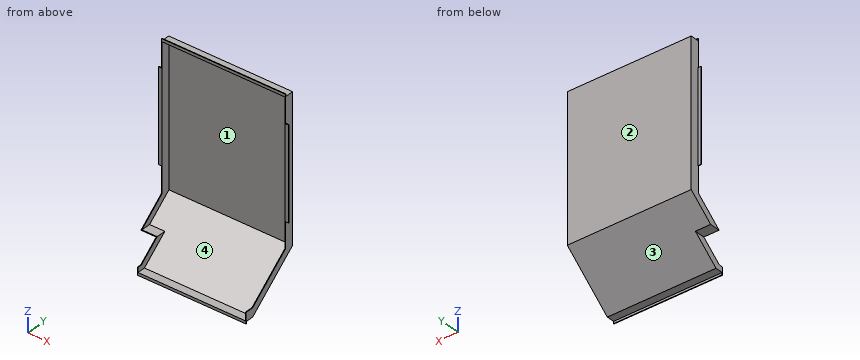
```python
from build123d import *

# Parameters (mm, degrees)
BOSS_EXTRUDE1_DEPTH  = 203
SKETCH4_W            = 2
SKETCH4_H            = 467.122613679
BOSS_EXTRUDE4_DEPTH  = 27
SKETCH5_W            = 2
SKETCH5_H            = 209.8319636
BOSS_EXTRUDE5_DEPTH  = 20
SKETCH6_W            = 2
SKETCH6_H            = 26.5
BOSS_EXTRUDE6_DEPTH  = 26.5
SKETCH14_W           = 300
SKETCH14_H           = 2
BOSS_EXTRUDE10_DEPTH = 10
SKETCH8_W            = 50
SKETCH8_H            = 77
CUT_EXTRUDE1_DEPTH   = 189.24061
BOSS_EXTRUDE7_DEPTH  = 48
SKETCH11_W           = 2
SKETCH11_H           = 107.789220226
BOSS_EXTRUDE8_DEPTH  = 20
CUT_EXTRUDE2_DEPTH   = 2
SKETCH13_W           = 2
SKETCH13_H           = 26.5
BOSS_EXTRUDE9_DEPTH  = 15.320889


with BuildPart() as part:
    # Sketch2 → Boss-Extrude1 (new body)
    with BuildSketch(Plane(origin=(0, 0, 0), x_dir=(0, 0, -1), z_dir=(1, 0, 0))):
        Polygon((-49.538744354, 1.5), (-49.538744354, -25.5), (-58.538744354, -25.5), (-58.538744354, -23.5), (-51.538744354, -23.5), (-51.538744354, 3.5), (418.516484641, 3.5), (554.461255643, -158.512669236), (554.461255643, -183.740609705), (561.461255643, -183.740609705), (561.461255643, -185.740609705), (552.461255643, -185.740609705), (552.461255643, -159.240609705), (417.583869325, 1.5), align=None)
    boss_extrude1 = extrude(amount=BOSS_EXTRUDE1_DEPTH)

    # Sketch4 → Boss-Extrude4 (add)
    with BuildSketch(Plane(origin=(0, 1.5, 0), x_dir=(-1, 0, 0), z_dir=(0, -1, 0))):
        with Locations((-202, 184.022562486)):
            Rectangle(SKETCH4_W, SKETCH4_H)
    boss_extrude4 = extrude(amount=BOSS_EXTRUDE4_DEPTH)

    # Sketch5 → Boss-Extrude5 (add)
    with BuildSketch(Plane(origin=(0, 206.239679889, -245.786879443), x_dir=(1, 0, 0), z_dir=(0, -0.6427876096865444, 0.7660444431189738))):
        with Locations((202, -372.184652342)):
            Rectangle(SKETCH5_W, SKETCH5_H)
    boss_extrude5 = extrude(amount=BOSS_EXTRUDE5_DEPTH)

    # Sketch6 → Boss-Extrude6 (add)
    with BuildSketch(Plane.XY.offset(-552.461255643)):
        with Locations((202, -172.490609705)):
            Rectangle(SKETCH6_W, SKETCH6_H)
    boss_extrude6 = extrude(amount=BOSS_EXTRUDE6_DEPTH)

    # Sketch14 → Boss-Extrude10 (add)
    with BuildSketch(Plane(origin=(203, 0, 0), x_dir=(0, 0, -1), z_dir=(1, 0, 0))):
        with Locations((181.461255646, -24.5)):
            Rectangle(SKETCH14_W, SKETCH14_H)
    boss_extrude10 = extrude(amount=BOSS_EXTRUDE10_DEPTH)

    # Mirror3: Boss-Extrude1, Boss-Extrude4, Boss-Extrude5, Boss-Extrude6, Boss-Extrude10 across plane
    add(boss_extrude1.mirror(Plane(origin=(0, 0, 0), x_dir=(0, 0, 1), z_dir=(1, 0, 0))))
    add(boss_extrude4.mirror(Plane(origin=(0, 0, 0), x_dir=(0, 0, 1), z_dir=(1, 0, 0))))
    add(boss_extrude5.mirror(Plane(origin=(0, 0, 0), x_dir=(0, 0, 1), z_dir=(1, 0, 0))))
    add(boss_extrude6.mirror(Plane(origin=(0, 0, 0), x_dir=(0, 0, 1), z_dir=(1, 0, 0))))
    add(boss_extrude10.mirror(Plane(origin=(0, 0, 0), x_dir=(0, 0, 1), z_dir=(1, 0, 0))))

    # Sketch8 → Cut-Extrude1 (cut)
    with BuildSketch(Plane(origin=(0, 3.5, 0), x_dir=(1, 0, 0), z_dir=(0, 1, 0))):
        with Locations((-178, 522.961255643)):
            Rectangle(SKETCH8_W, SKETCH8_H)
    extrude(amount=-CUT_EXTRUDE1_DEPTH, mode=Mode.SUBTRACT)

    # Sketch10 → Boss-Extrude7 (add)
    with BuildSketch(Plane(origin=(-201, 0, 0), x_dir=(0, 0, -1), z_dir=(1, 0, 0))):
        Polygon((484.461255643, -109.315841945), (484.461255643, -78.201365408), (483.175680424, -76.669276522), (483.175680424, -107.783753059), align=None)
    extrude(amount=BOSS_EXTRUDE7_DEPTH)

    # Sketch11 → Boss-Extrude8 (add)
    with BuildSketch(Plane(origin=(0, 206.239679889, -245.786879443), x_dir=(1, 0, 0), z_dir=(0, -0.6427876096865444, 0.7660444431189738))):
        with Locations((-152, -423.206024029)):
            Rectangle(SKETCH11_W, SKETCH11_H)
    extrude(amount=BOSS_EXTRUDE8_DEPTH)

    # Sketch12 → Cut-Extrude2 (cut)
    with BuildSketch(Plane.ZY.offset(153)):
        Polygon((-483.175680424, -76.669276522), (-483.175680424, -107.783753059), (-467.854791561, -89.525028716), align=None)
    extrude(amount=-CUT_EXTRUDE2_DEPTH, mode=Mode.SUBTRACT)

    # Sketch13 → Boss-Extrude9 (add)
    with BuildSketch(Plane.XY.offset(-552.461255643)):
        with Locations((-152, -172.490609705)):
            Rectangle(SKETCH13_W, SKETCH13_H)
    extrude(amount=BOSS_EXTRUDE9_DEPTH)


solid = part.part
```
CAD build for the part. Positions are in the model's coordinates, mm. Face numbers are marked on the shaded views. A direction names the side the tool comes from. Coordinates: 2 decimals unless noted, no trailing zeros. Write each loop counter-clockwise with the first axis right and the second up, starting at its lowest first coordinate (ties: lowest second). Pieces come first, ordered by that corner, then holes. Notation, with made-up numbers: (43.5, -16) -> (49.5, -16) arc R16 ccw to (49.5, 5) -> close; hole circle Ø8 at (54.5, 10). An arc over 180 degrees is marked (long way). Use CSV: the item, a comma, the result in double quotes. Start each with the question number.
Item 1: Band-saw the part on C-C, the plane y = -100.5. Write the cut outline in (x, z), plus the area to 3 significant figures.
Item 2: Drop flat-ended pins along their axis: P1, Ø13.5, axis at x = -12.5, y = -17.5, coming from the -Z side; P2, Ø25, axis at x = -184.5, y = -90.5, coming from the +Z side; P3, Ø10, axis at x = 18, y = -52, coming from the -Z side. Give the stop position or say it passes through.
Item 3: Band-saw the part on A-A, the plane z = -378. Write the cut outline in (x, y), plus the area to 3 significant figures.
Item 4: Two-plate mould, pull along X, no slides. Class the marked faces 3 and 4: +X half, -X half, draft (parallel to the pull), parting line (faces both ways), or undercut.
Item 5: Tool access for the marked faces 1 and 2: list every direction of +Z, -Z, +X, -X, +Y, -Y with a clear straight run to the whole face (end or side of a thin tool).
Item 6: Band-saw the part on B-B, the plane x = -68.5. Write the cut outline in (y, z).
Item 7: Wall check: probe 1 along X at (y, z) = (-21, -108); probe 2 along Y at (x, z) = (17.5, -334); probe 3 along Z at (x, y) = (-86, -8). Give the ranges that are in metal, low to high.
Item 8: Band-saw the part on D-D, the plane x = -182. Write the cut outline in (y, z), plus the area to 3 significant figures.
Response values:
1,outline,"(-203, -484.46) -> (-153, -484.46) -> (-153, -505.78) -> (203, -505.78) -> (203, -477.06) -> (201, -477.06) -> (201, -503.17) -> (-151, -503.17) -> (-151, -483.18) -> (-201, -483.18) -> (-201, -477.06) -> (-203, -477.06) -> close"
1,area,"1,100 mm2"
2,P1,"stops at z = -441.8"
2,P2,"stops at z = -483.18"
2,P3,"stops at z = -469.28"
3,outline,"(-203, -25.5) -> (-201, -25.5) -> (-201, 1.5) -> (201, 1.5) -> (201, -25.5) -> (203, -25.5) -> (203, 3.5) -> (-203, 3.5) -> close"
3,area,"920 mm2"
4,face 3,"draft"
4,face 4,"undercut"
5,face 1,"-Y"
5,face 2,"+Z, -Z, +X, -X, +Y"
6,outline,"(-185.74, -561.46) -> (-183.74, -561.46) -> (-183.74, -554.46) -> (-158.51, -554.46) -> (3.5, -418.52) -> (3.5, 51.54) -> (-23.5, 51.54) -> (-23.5, 58.54) -> (-25.5, 58.54) -> (-25.5, 49.54) -> (1.5, 49.54) -> (1.5, -417.58) -> (-159.24, -552.46) -> (-185.74, -552.46) -> close"
7,probe 1,"x = -203 to -201, 201 to 203"
7,probe 2,"y = 1.5 to 3.5"
7,probe 3,"z = -428.17 to -425.56, 49.54 to 51.54"
8,outline,"(-109.32, -484.46) -> (-75.09, -484.46) -> (3.5, -418.52) -> (3.5, 51.54) -> (-23.5, 51.54) -> (-23.5, 58.54) -> (-25.5, 58.54) -> (-25.5, 49.54) -> (1.5, 49.54) -> (1.5, -417.58) -> (-76.67, -483.18) -> (-107.78, -483.18) -> close"
8,area,"1,250 mm2"
